```python
from build123d import *

# Parameters (mm, degrees)
F1_DEPTH = 20
F2_R     = 3
F3_DEPTH = 25
F4_R     = 3
F5_DEPTH = 25


with BuildPart() as f1:
    # F0 (on Front) → F1 (new body)
    with BuildSketch(Plane.XZ):
        Polygon((0, 90), (0, 0), (90, 0), (90, 30), (80, 30), (30, 80), (30, 90), align=None)
    extrude(amount=F1_DEPTH)

    # F2 (on face) → F3 (cut)
    with BuildSketch(Plane(origin=(0, 0, 0), x_dir=(0, -1, 0), z_dir=(-1, 0, 0))):
        with Locations((10, 20)):
            Circle(F2_R)
        with Locations((10, 45)):
            Circle(F2_R)
        with Locations((10, 80)):
            Circle(F2_R)
    extrude(amount=-F3_DEPTH, mode=Mode.SUBTRACT)

    # F4 (on face) → F5 (cut)
    with BuildSketch(Plane(origin=(0, 0, 0), x_dir=(1, 0, 0), z_dir=(0, 0, -1))):
        with Locations((20, 10)):
            Circle(F4_R)
        with Locations((45, 10)):
            Circle(F4_R)
        with Locations((80, 10)):
            Circle(F4_R)
    extrude(amount=-F5_DEPTH, mode=Mode.SUBTRACT)


solid = f1.part
```
Build history of the part. All positions in model axes, mm. A direction names the side the tool comes from. Give positions to 0.01 mm unless a question says otherwise; leave off trailing zeros. Loops run counter-clockwise (first coordinate to the right, second up) from the corner with the lowest first, then second, coordinate; pieces in that order, holes last.
1) Drop flat-ended pins along their axis: P1, Ø7, axis at y = -10, z = 45, coming from the -X side; P2, Ø3, axis at x = 20.5, y = -11, coming from the -Z side; P3, Ø4, axis at y = -16, z = 39.5, coming from the +X side; P4, Ø1.8, axis at y = -11, z = 79.5, coming from the -X side. Give the stop position or say it passes through.
Values follow:
P1: stops at x = 0
P2: stops at z = 25
P3: stops at x = 72.5
P4: stops at x = 25
2) Band-saw the part on C-C on z = 34. List the corners of the cut face in (x, y), then the cut area to 3 significant figures.
Values follow:
outline: (0, -20) - (76, -20) - (76, 0) - (0, 0) - close
area: 1,520 mm2
3) 3-axis set-ups, long thin cutter, end or side, ignore diameter. For faces 4 (the face through (85, -10, 30)), 5 (the face through (23, -7.6, 18.2)), 6 (the face through (80, -10, 25)): which of +Z, -Z, +X, -X, +Y, -Y reach the whole face in a straight line?
Values follow:
face 4: +Z, +X, +Y, -Y
face 5: -X
face 6: -Z
4) Band-saw the part on A-A on x = 13.5. List the corners of the cut face in (y, z).
Values follow:
outline: (-20, 0) - (0, 0) - (0, 90) - (-20, 90) - close; hole circle Ø6 at (-10, 20); hole circle Ø6 at (-10, 45); hole circle Ø6 at (-10, 80)
5) Two-plate mould, pull along X, no slides. Class faces 1 (the face through (17, -10, 10)), 2 (the face through (12.32, -9.35, 77.07)), 3 (the face through (30, -10, 85)): released by +X, released by -X, zero draft, split by the parting line, or undercut.
Values follow:
face 1: undercut
face 2: zero draft
face 3: released by +X
6) Band-saw the part on B-B on y = -3.75. List the corners of the cut face in (x, z), then the cut area to 3 significant figures.
Values follow:
outline: (0, 0) - (90, 0) - (90, 30) - (80, 30) - (30, 80) - (30, 90) - (0, 90) - close
area: 5,750 mm2
7) Probe line 1 along Z through (x, y) = (23.4, -10); line 2 along Z through (x, y) = (18.5, -10). List the from-to ranges inside material, lowest first.
Values follow:
line 1: z = 0 to 17, 23 to 42, 48 to 77, 83 to 90
line 2: z = 25 to 42, 48 to 77, 83 to 90
8) Band-saw the part on D-D on x = 74. List the corners of the cut face in (y, z), then the cut area to 3 significant figures.
Values follow:
outline: (-20, 0) - (0, 0) - (0, 36) - (-20, 36) - close
area: 720 mm2
